Read the model definition and answer for the solid it produces. Units are mm, in the model's axes. Face numbers are marked on the shaded views. A direction names the side the tool comes from. Give positions to 0.01 mm unless a question says otherwise; leave off trailing zeros. Order: outer loops, then holes, each group sorted by start corner. A loop starts at its lowest first (then second) coordinate and runs counter-clockwise, first axis right, second up. Notation, with made-up numbers: (2.25, 30.25) -> (6.25, 30.25) arc R17 cw to (6.25, 36.25) -> close; hole circle Ø2 at (-29.75, 72). An arc over 180 degrees is marked (long way). Use one line per item in the form item = value.
```python
from build123d import *

# Parameters (mm, degrees)
F1_DEPTH = 2
F0_W     = 26
F0_H     = 20
F2_DEPTH = 30
F3_W     = 26
F3_H     = 20
F4_DEPTH = 10
F5_W     = 7
F5_H     = 15
F6_DEPTH = 2


with BuildPart() as f1:
    # F0 (on Top) → F1 (new body)
    with BuildSketch(Plane.XY):
        Polygon((20, -20), (20, 20), (-20, 20), (-20, -20), (-13, -20), (-13, 0), (13, 0), (13, -20), align=None)
    extrude(amount=F1_DEPTH)



with BuildPart() as f2:
    # F0 (on Top) → F2 (new body)
    with BuildSketch(Plane.XY):
        with Locations((0, -10)):
            Rectangle(F0_W, F0_H)
    extrude(amount=F2_DEPTH)


with BuildPart() as f1_1:
    add(f1.part)

    add(f2.part)  # F4 merges F2
    # F3 (on face) → F4 (join)
    with BuildSketch(Plane.XY.offset(2)):
        with Locations((0, 10)):
            Rectangle(F3_W, F3_H)
    extrude(amount=F4_DEPTH)

    # F5 (on face) → F6 (join)
    with BuildSketch(Plane.XY.offset(2)):
        with Locations((16.5, -7.5)):
            Rectangle(F5_W, F5_H)
        with Locations((-16.5, -7.5)):
            Rectangle(F5_W, F5_H)
    extrude(amount=F6_DEPTH)


solid = f1_1.part
```
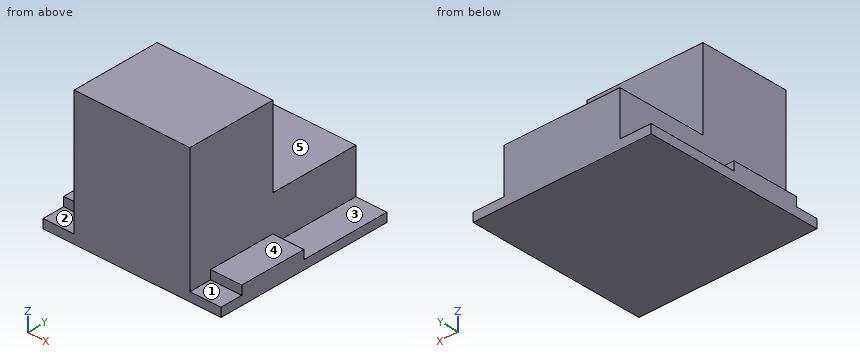
Item 1: The part is cut by section D-D on x = -10.5. Give the vertices of the cut face in (y, z), and give its area (3 significant figures).
Checks:
outline = (-20, 0) -> (20, 0) -> (20, 12) -> (0, 12) -> (0, 30) -> (-20, 30) -> close
area = 840 mm²
Item 2: Which of the six approach directions +Z, -Z, +X, -X, +Y, -Y give full straight-line access (tool end or side, diameter ignored) to the marked faces 1, 2, 3, 4 and 5?
Checks:
face_1 = +Z, +X, -Y
face_2 = +Z, -X, -Y
face_3 = +Z, +X, +Y
face_4 = +Z, +X, +Y, -Y
face_5 = +Z, +X, -X, +Y
Item 3: Straight lines are drawn through the part: L1, parallel to Y at x = 12.5, z = 26.5; L2, parallel to Z at x = -16, y = -11.5; L3, parallel to X at y = -4.5, z = 17.5. For each, find the intervals that lie inside material, in ascending order. Write a range as from..to.
Checks:
L1 = -20..0
L2 = 0..4
L3 = -13..13
Item 4: The part is cut by section A-A on x = -15. Give the vertices of the cut face in (y, z).
Checks:
outline = (-20, 0) -> (20, 0) -> (20, 2) -> (0, 2) -> (0, 4) -> (-15, 4) -> (-15, 2) -> (-20, 2) -> close
Item 5: The part is cut by section B-B on y = 2. Give the vertices of the cut face in (x, z).
Checks:
outline = (-20, 0) -> (20, 0) -> (20, 2) -> (13, 2) -> (13, 12) -> (-13, 12) -> (-13, 2) -> (-20, 2) -> close
Item 6: The part is cut by section C-C on z = 23.5. Give the vertices of the cut face in (x, y), and give its area (3 significant figures).
Checks:
outline = (-13, -20) -> (13, -20) -> (13, 0) -> (-13, 0) -> close
area = 520 mm²
Item 7: Given pin 1 Ø8.5 at (y, z) = (-9, 10.5) entering from -X; pin 2 Ø7.5 at (x, y) = (16.5, 13.5) entering from +Z; pin 3 Ø2 at (x, y) = (-16.5, 13.5) entering from +Z, each flat-ended and moving along its own axis, determine where each tip first touches the part or whether it passes through.
Checks:
pin_1 = -13
pin_2 = 12
pin_3 = 2
